Source: CAD feature listing. Evaluate the final solid. Frame: model axes, mm. Round coordinates to 2 decimals unless told otherwise and drop trailing zeros. Write each loop counter-clockwise with the first axis right and the second up, starting at its lowest first coordinate (ties: lowest second). Pieces come first, ordered by that corner, then holes. Notation, with made-up numbers: (-26, 79.25) -> (-11, 79.25) arc R32 cw to (-11, 114.25) -> close; hole circle Ø10 at (28, 73). An arc over 180 degrees is marked (long way). Put each result on its own line as item: value.
```python
from build123d import *

# Parameters (mm, degrees)
SKETCH1_R           = 1.778
BOSS_EXTRUDE1_DEPTH = 6.35
SKETCH2_W           = 10.758447183
SKETCH2_H           = 9.8425
CUT_EXTRUDE1_DEPTH  = 84.373202748


with BuildPart() as part:
    # Sketch1 → Boss-Extrude1 (new body)
    with BuildSketch(Plane(origin=(0, 6.35, 0), x_dir=(1, 0, 0), z_dir=(0, 1, 0))):
        with BuildLine():
            Line((78.232, 4.7625), (-78.232, 4.7625))
            ThreePointArc((-78.232, 4.7625), (-82.9945, 0), (-78.232, -4.7625))
            Line((-78.232, -4.7625), (78.232, -4.7625))
            ThreePointArc((78.232, -4.7625), (82.9945, 0), (78.232, 4.7625))
        make_face()
        with Locations(Location((78.232, 0, 0), (0, 0, 90))):
            Circle(SKETCH1_R, mode=Mode.SUBTRACT)
        with Locations(Location((68.453, 0, 0), (0, 0, 90))):
            Circle(SKETCH1_R, mode=Mode.SUBTRACT)
        with Locations(Location((58.674, 0, 0), (0, 0, 90))):
            Circle(SKETCH1_R, mode=Mode.SUBTRACT)
        with Locations(Location((48.895, 0, 0), (0, 0, 90))):
            Circle(SKETCH1_R, mode=Mode.SUBTRACT)
        with Locations(Location((39.116, 0, 0), (0, 0, 90))):
            Circle(SKETCH1_R, mode=Mode.SUBTRACT)
        with Locations(Location((29.337, 0, 0), (0, 0, 90))):
            Circle(SKETCH1_R, mode=Mode.SUBTRACT)
        with Locations(Location((19.558, 0, 0), (0, 0, 90))):
            Circle(SKETCH1_R, mode=Mode.SUBTRACT)
        with Locations(Location((9.779, 0, 0), (0, 0, 90))):
            Circle(SKETCH1_R, mode=Mode.SUBTRACT)
        with Locations(Location((0, 0, 0), (0, 0, 90))):
            Circle(SKETCH1_R, mode=Mode.SUBTRACT)
        with Locations(Location((-9.779, 0, 0), (0, 0, 90))):
            Circle(SKETCH1_R, mode=Mode.SUBTRACT)
        with Locations(Location((-19.558, 0, 0), (0, 0, 90))):
            Circle(SKETCH1_R, mode=Mode.SUBTRACT)
        with Locations(Location((-29.337, 0, 0), (0, 0, 90))):
            Circle(SKETCH1_R, mode=Mode.SUBTRACT)
        with Locations(Location((-39.116, 0, 0), (0, 0, 90))):
            Circle(SKETCH1_R, mode=Mode.SUBTRACT)
        with Locations(Location((-48.895, 0, 0), (0, 0, 90))):
            Circle(SKETCH1_R, mode=Mode.SUBTRACT)
        with Locations(Location((-58.674, 0, 0), (0, 0, 90))):
            Circle(SKETCH1_R, mode=Mode.SUBTRACT)
        with Locations(Location((-68.453, 0, 0), (0, 0, 90))):
            Circle(SKETCH1_R, mode=Mode.SUBTRACT)
        with Locations(Location((-78.232, 0, 0), (0, 0, 90))):
            Circle(SKETCH1_R, mode=Mode.SUBTRACT)
    extrude(amount=-BOSS_EXTRUDE1_DEPTH)

    # Sketch2 → Cut-Extrude1 (cut, through all)
    with BuildSketch(Plane(origin=(0, 6.35, 0), x_dir=(1, 0, 0), z_dir=(0, 1, 0))):
        with Locations((-77.642223591, 0.15875)):
            Rectangle(SKETCH2_W, SKETCH2_H)
    extrude(amount=-CUT_EXTRUDE1_DEPTH, mode=Mode.SUBTRACT)


solid = part.part
```
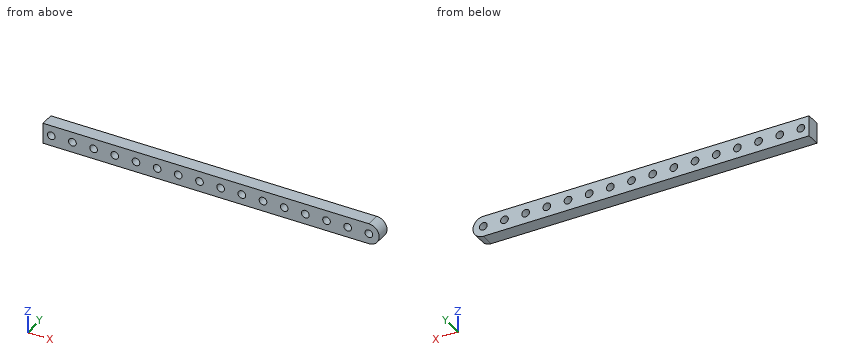
Q1. Cut plane A-A on x = 0. Output: boundary loops of the cut face in (y, z).
Ans:
outline: (0, -4.76) -> (6.35, -4.76) -> (6.35, -1.78) -> (0, -1.78) -> close; (0, 1.78) -> (6.35, 1.78) -> (6.35, 4.76) -> (0, 4.76) -> close
Q2. Material intervals for line 1 (Z direction, x = 49, y = 3.75); line 2 (Z direction, x = 69, y = 2.5); line 3 (X direction, y = 1.25, z = -2.75), sorted ascending. Write a range as [from, to].
Ans:
line 1: z = [-4.76, -1.77], [1.77, 4.76]
line 2: z = [-4.76, -1.69], [1.69, 4.76]
line 3: x = [-72.26, 82.12]
Q3. Cut plane B-B on y = 3. Give the number of separate pieces and of enclosed holes in the cut face, and give its area (3 significant figures).
Ans:
separate pieces: 1
enclosed holes: 16
area: 1,310 mm^2
